The listing builds one solid part. Answer for the finished solid, in the listing's coordinates (mm). A direction names the side the tool comes from. Coordinates: 2 decimals unless noted, no trailing zeros. Loops run counter-clockwise (first coordinate to the right, second up) from the corner with the lowest first, then second, coordinate; pieces in that order, holes last. Notation, with made-up numbers: (11, -17) - (40, -17) arc R27 ccw to (40, 11) - close; hole circle Ø2 at (-23, 49). An arc over 180 degrees is marked (long way). One line per question, with ' | ' between items.
from build123d import *

# Parameters (mm, degrees)
BOSS_EXTRUDE1_DEPTH      = 15
FILLET1_R                = 20
FILLET2_R                = 15
BOSS_EXTRUDE2_DEPTH      = 25
BOSS_EXTRUDE2_DEPTH_BACK = 21
SKETCH2_W                = 5
SKETCH2_H                = 60
CUT_EXTRUDE1_DEPTH       = 5
CUT_EXTRUDE2_DEPTH       = 62


with BuildPart() as part:
    # Sketch1 → Boss-Extrude1 (new body)
    # profile 1 of 6: a face of its own
    with BuildSketch(Plane.XY):
        with BuildLine():
            Line((-20, -30), (-30, -30))
            ThreePointArc((-30, -30), (-29.388396861, -36.026784376), (-27.578524672, -41.807835403))
            Line((-27.578524672, -41.807835403), (-20, -30))
        make_face()
    # profile 2 of 6: a face of its own
    with BuildSketch(Plane.XY):
        with BuildLine():
            Line((0, -10), (0, 0))
            ThreePointArc((0, 0), (-21.213203436, -8.786796564), (-30, -30))
            Line((-30, -30), (-20, -30))
            ThreePointArc((-20, -30), (-14.142135624, -15.857864376), (0, -10))
        make_face()
    # profile 3 of 6: a face of its own
    with BuildSketch(Plane.XY):
        with BuildLine():
            ThreePointArc((0, -50), (-14.142135624, -44.142135624), (-20, -30))
            Line((-20, -30), (-27.578524672, -41.807835403))
            ThreePointArc((-27.578524672, -41.807835403), (-16.519154608, -55.04231481), (0, -60))
            Line((0, -60), (0, -50))
        make_face()
    # profile 4 of 6: a face of its own
    with BuildSketch(Plane.XY):
        with BuildLine():
            ThreePointArc((-27.578524672, -41.807835403), (-29.388396861, -36.026784376), (-30, -30))
            Line((-30, -30), (-49.254650189, -60))
            Line((-49.254650189, -60), (-30, -105))
            ThreePointArc((-30, -105), (-28.650020621, -98.780921528), (-24.84307506, -93.681260081))
            Line((-24.84307506, -93.681260081), (-39.254650189, -60))
            Line((-39.254650189, -60), (-27.578524672, -41.807835403))
        make_face()
    # profile 5 of 6: a face of its own
    with BuildSketch(Plane.XY):
        with BuildLine():
            ThreePointArc((-24.84307506, -93.681260081), (-28.650020621, -98.780921528), (-30, -105))
            Line((-30, -105), (-20, -105))
            Line((-20, -105), (-24.84307506, -93.681260081))
        make_face()
    # profile 6 of 6: a face of its own
    with BuildSketch(Plane.XY):
        with BuildLine():
            Line((-20, -105), (-30, -105))
            ThreePointArc((-30, -105), (-15, -120), (0, -105))
            ThreePointArc((0, -105), (-8.780921528, -91.349979379), (-24.84307506, -93.681260081))
            Line((-24.84307506, -93.681260081), (-20, -105))
        make_face()
        with BuildLine():
            ThreePointArc((-10, -105), (-15, -110), (-20, -105))
            ThreePointArc((-20, -105), (-15, -100), (-10, -105))
        make_face(mode=Mode.SUBTRACT)
    extrude(amount=BOSS_EXTRUDE1_DEPTH)

    # Fillet1
    fillet1_edges = [part.edges().sort_by_distance(p)[0] for p in [
        (-39.254650189, -60, 7.5),
        (-49.254650189, -60, 7.5),
    ]]
    fillet(fillet1_edges, radius=FILLET1_R)

    # Fillet2
    # the kernel refuses this fillet: 15 mm, written as the material it takes off along each edge
    with BuildSketch(Plane(origin=(0, -50, -25), x_dir=(-0.9759000729485309, 0.21821789023600283, 0), z_dir=(0, 0, 1))) as fillet2_piece_1:
        with BuildLine():
            CenterArc((12.001983963, 14.638501094), FILLET2_R, 198.983752857, 58.411864495)
            Line((-2.182178902, 9.759000729), (-2.46586216, 9.661410722))
            ThreePointArc((-2.46586216, 9.661410722), (-1.383859473, 4.814034998), (-0.292770022, -0.065465367))
            Line((-0.292770022, -0.065465367), (0.065465367, -0.292770022))
            ThreePointArc((0.065465367, -0.292770022), (4.364357805, 0.181998541), (8.663250242, -0.292770022))
            Line((8.663250242, -0.292770022), (8.728715609, 0))
        make_face()
    extrude(amount=65, mode=Mode.SUBTRACT)
    with BuildSketch(Plane(origin=(0, -10, -25), x_dir=(0, 1, 0), z_dir=(0, 0, 1))) as fillet2_piece_2:
        with BuildLine():
            CenterArc((11.666666667, 14.90711985), FILLET2_R, 205.208765297, 58.411864495)
            Line((-1.904761905, 8.5183542), (-2.176190476, 8.390578887))
            ThreePointArc((-2.176190476, 8.390578887), (-0.774768563, 4.298892438), (-0.3, 0))
            Line((-0.3, 0), (0, -0.3))
            ThreePointArc((0, -0.3), (5, -0.3), (9.966666667, -0.298142397))
            Line((9.966666667, -0.298142397), (10, 0))
        make_face()
    extrude(amount=65, mode=Mode.SUBTRACT)

    # Sketch2 → Boss-Extrude2 (add, two sides: drawn at the far end of the back side and taken through both)
    with BuildSketch(Plane(origin=(0, 0, 0), x_dir=(0, 0, -1), z_dir=(1, 0, 0)).offset(-BOSS_EXTRUDE2_DEPTH_BACK)):
        with Locations((-7.5, -30)):
            Rectangle(SKETCH2_W, SKETCH2_H)
    extrude(amount=BOSS_EXTRUDE2_DEPTH + BOSS_EXTRUDE2_DEPTH_BACK)

    # Sketch3 → Cut-Extrude1 (cut)
    with BuildSketch(Plane(origin=(0, 0, 5), x_dir=(-1, 0, 0), z_dir=(0, 0, -1))):
        with BuildLine():
            Line((0, 0), (-25, 0))
            Line((-25, 0), (-25, -30.000000042))
            ThreePointArc((-25, -30.000000042), (-17.141969276, -11.802393307), (1.49223119, -5.044574817))
            ThreePointArc((1.49223119, -5.044574817), (0.523240843, -2.588215791), (0, 0))
        make_face()
        with BuildLine():
            Line((21, 0), (0, 0))
            ThreePointArc((0, 0), (11.341768853, -2.226554422), (21, -8.575714714))
            Line((21, -8.575714714), (21, 0))
        make_face()
        with BuildLine():
            ThreePointArc((1.49223119, -54.955425183), (-17.141969245, -48.197606722), (-25, -30.000000042))
            Line((-25, -30.000000042), (-25, -60))
            Line((-25, -60), (0, -60))
            ThreePointArc((0, -60), (0.523240843, -57.411784209), (1.49223119, -54.955425183))
        make_face()
        with BuildLine():
            ThreePointArc((21, -51.424285286), (11.341768853, -57.773445578), (0, -60))
            Line((0, -60), (21, -60))
            Line((21, -60), (21, -51.424285286))
        make_face()
    extrude(amount=-CUT_EXTRUDE1_DEPTH, mode=Mode.SUBTRACT)

    # Sketch4 → Cut-Extrude2 (cut)
    with BuildSketch(Plane(origin=(0, 0, 0), x_dir=(1, 0, 0), z_dir=(0, 1, 0))):
        Polygon((0, -5), (25, -7.5), (25, -5), align=None)
        Polygon((25, -10), (25, -7.5), (0, -10), align=None)
    extrude(amount=-CUT_EXTRUDE2_DEPTH, mode=Mode.SUBTRACT)


solid = part.part
Item 1: Find section B-B, the plane x = -15. Write down the section's boundary in (y, z).
Taken from the geometry:
outline: (-120, 0) - (-110, 0) - (-110, 15) - (-120, 15) - close; (-100, 0) - (-90, 0) - (-90, 15) - (-100, 15) - close; (-55.98, 0) - (-43.23, 0) - (-43.23, 5) - (-16.77, 5) - (-16.77, 0) - (-4.02, 0) - (-4.02, 15) - (-16.77, 15) - (-16.77, 10) - (-43.23, 10) - (-43.23, 15) - (-55.98, 15) - close
Item 2: Which of the six approach directions +Z, -Z, +X, -X, +Y, -Y give full straight-line access (tool end or side, diameter ignored) to faces 1 (the face through (-8, -30, 10)), 2 (the face through (-34.1, -72.5, 0)), 3 (the face through (-36.64, -60.36, 7.6))?
Taken from the geometry:
face 1: +Z, +X | face 2: -Z, +X, -X, +Y, -Y | face 3: +Z, -Z
Item 3: Find section D-D, the plane x = -40. Write down the section's boundary in (y, z).
Taken from the geometry:
outline: (-81.63, 0) - (-45.58, 0) - (-45.58, 15) - (-81.63, 15) - close
Item 4: The mould has two halves that part along Y. Classify faces 4 (the face through (-46.64, -60.36, 7.6)), 5 (the face through (-37.647, -87.127, 7.395)), 6 (the face through (-8, -30, 5)): pulls with the +Y half, pulls with the -Y half, needs draft (parallel to the pull), parting line crosses it, or undercut.
Taken from the geometry:
face 4: parting line crosses it | face 5: pulls with the -Y half | face 6: undercut
Item 5: Find the intervals of material crossed by line 1 (Y direction, x = -15, z = 4.25); line 2 (Y direction, x = -15, z = 8.25); line 3 (Y direction, x = -1.5, z = 1.5), in increasing order. Write a range as [from, to].
Taken from the geometry:
line 1: y = [-120, -110], [-100, -90], [-55.98, -43.23], [-16.77, -4.02] | line 2: y = [-120, -110], [-100, -90], [-55.98, -4.02] | line 3: y = [-111.54, -98.46], [-59.96, -54.94], [-5.06, -0.04]
Item 6: Find section A-A, the plane x = -3. Write down the section's boundary in (y, z), plus the area to 3 significant figures.
Taken from the geometry:
outline: (-114, 0) - (-96, 0) - (-96, 15) - (-114, 15) - close; (-59.85, 0) - (-52.54, 0) - (-52.54, 5) - (-7.46, 5) - (-7.46, 0) - (-0.15, 0) - (-0.15, 15) - (-7.46, 15) - (-7.46, 10) - (-52.54, 10) - (-52.54, 15) - (-59.85, 15) - close | area: 715 mm2
Item 7: Each of these flat-tipped pins is pushed along its axis until it touches: pin 1 Ø4 at (y, z) = (-16, 13) entering from +X; pin 2 Ø2 at (x, y) = (15, -28) entering from -Z; pin 3 Ø1.5 at (y, z) = (-82, 12) entering from -X; pin 4 Ø12 at (x, y) = (-2, -50.5) entering from -Z. Where does it stop, or does it pass through?
Taken from the geometry:
pin 1: stops at x = -12 | pin 2: stops at z = 6.4 | pin 3: stops at x = -40.16 | pin 4: stops at z = 0
